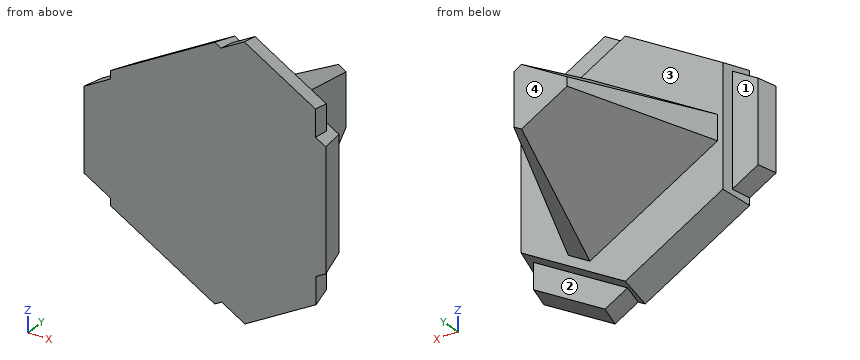
```python
from build123d import *

# Parameters (mm, degrees)
PATTERN_CIRCULAR_1_COUNT = 3


with BuildPart() as part:
    # 草图4 → 放样5 section 0
    with BuildSketch(Plane(origin=(0, 200, 0), x_dir=(1, 0, 0), z_dir=(0, 1, 0))):
        Polygon((0, 793.295), (-664.472424785, 409.655), (-664.472424785, -409.655), (0, -793.295), (709.5403868, -383.635), (709.5403868, 383.635), align=None)
    # 草图1 → 放样5 section 1
    with BuildSketch(Plane(origin=(0, 0, 0), x_dir=(1, 0, 0), z_dir=(0, 1, 0))):
        Polygon((-710.882424785, -436.449593178), (-1.2807e-05, -846.88487741), (755.9503868, -410.429607966), (755.9503868, 410.429607966), (-1.2807e-05, 846.88487741), (-710.882424785, 436.449593178), align=None)
    loft()

    # 草图8 → 放样8 section 0
    with BuildSketch(Plane(origin=(0, 130.08, 0), x_dir=(1, 0, 0), z_dir=(0, 1, 0))):
        Polygon((-676.032424785, 384.41), (-676.032424785, -384.41), (-856.59006122, -280.165), (-856.59006122, 280.165), align=None)
    # 草图7 → 放样8 section 1
    with BuildSketch(Plane(origin=(0, 0, 0), x_dir=(1, 0, 0), z_dir=(0, 1, 0))):
        Polygon((-710.882424785, 387.274170973), (-891.44006122, 283.029170973), (-891.44006122, -277.300829027), (-710.882424785, -381.545829027), align=None)
    loft_8 = loft()

    # 阵列(圆周)1: 放样8 ×3 about axis
    pattern_circular_1_axis = Axis((0, 0, 0), (0, 1, 0))
    for i in range(1, PATTERN_CIRCULAR_1_COUNT):
        add(loft_8.rotate(pattern_circular_1_axis, i * 360 / PATTERN_CIRCULAR_1_COUNT))

    # 草图11 → 放样9 section 0
    with BuildSketch(Plane(origin=(0, 1111.8, 0), x_dir=(1, 0, 0), z_dir=(0, 1, 0))):
        Polygon((-223.984859664, 30.416313823), (-223.984859664, -30.413899524), (85.653863205, -209.183899524), (138.334158952, -178.768421621), (138.334158952, 178.771578379), (85.653648875, 209.186685053), align=None)
    # 草图10 → 放样9 section 1
    with BuildSketch(Plane(origin=(0, 200, 0), x_dir=(1, 0, 0), z_dir=(0, 1, 0))):
        Polygon((240.301512133, 586.87442815), (388.097407543, 501.54442815), (388.097407543, -501.53557185), (240.30211344, -586.866613336), (-628.39064859, -85.32661334), (-628.39064859, 85.33338666), align=None)
    loft()


solid = part.part
```
Work out the finished part from the listing and answer in its coordinate system (mm). Face numbers are marked on the shaded views. A direction names the side the tool comes from. Round coordinates to 2 decimals unless told otherwise and drop trailing zeros.
(1) For the marked faces 1, 2, 3 and 4, determine the directions among +Z, -Z, +X, -X, +Y, -Y from which every point of the face is accessible in a straight line to the end or side of a thin tool.
Computed values:
face 1: +Z, -Z, -X, +Y
face 2: -Z, +X, +Y
face 3: +Y
face 4: +Z, -Z, +X, -X, +Y
(2) Each of these flat-tipped pins is pushed along its axis until it touches: P1, Ø4, axis at x = -367, z = 257.5, coming from the +Y side; P2, Ø3, axis at x = -581.5, y = 288, coming from the -Z side; P3, Ø12, axis at x = -515.5, y = 169.5, coming from the +Z side. Where does it stop, or does it pass through?
Computed values:
P1: stops at y = 200
P2: stops at z = -85.56
P3: stops at z = 507.66
(3) Find the intervals of material crossed by L1, parallel to Y at x = 467, z = 314; L2, parallel to Z at x = -35.5, y = 336; L3, parallel to X at y = 215, z = 87, in increasing order.
Computed values:
L1: y = 0 to 200
L2: z = -384.62 to 384.62
L3: x = -617.27 to 383.99
